Autodesk Inventor part; units mm, degrees
ref_plane "YZ Plane" through (0, 0, 0) normal (1, 0, 0) x (0, 1, 0)
ref_plane "XZ Plane" through (0, 0, 0) normal (0, 1, 0) x (-1, 0, 0)
ref_plane "XY Plane" through (0, 0, 0) normal (0, 0, 1) x (1, 0, 0)
sketch "Sketch1" plane through (0, 0, 0) normal (1, 0, 0) x (0, 1, 0)
  line L0 (-15.866, 25.4808) -> (14.134, -26.4808)
  line L1 (14.134, -26.4808) -> (15.866, -25.4808)
  line L2 (15.866, -25.4808) -> (-14.134, 26.4808)
  line L3 (-14.134, 26.4808) -> (-15.866, 25.4808)
  line L4 (-15.866, 25.4808) -> (15.866, -25.4808) construction
  line L5 (14.134, -26.4808) -> (-14.134, 26.4808) construction
  line L6 (-15.866, 25.4808) -> (44.134, 25.4808) construction
  point P0 (0, 0)
  dimension "d0" = 60
  dimension "d1" = 60
  dimension "d2" = 2
extrude "Extrusion1" add sketch "Sketch1" along normal blind 150
sketch "Sketch2" plane through (0, 0, 0) normal (0, 1, 0) x (-1, 0, 0)
  circle A0 centre (0, 0) radius 16.75
  dimension "d5" = 33.5
extrude "Extrusion2" cut sketch "Sketch2" along normal through all both and the other way through all
fillet "Fillet1" radius 2 4 edges at (150, -15, 25.9808) (150, 15, -25.9808) (0, -15, 25.9808) (0, 15, -25.9808)
equation "\"BendRadius\" = Thickness"
equation "\"BendReliefWidth\" = Thickness"
equation "\"BendReliefDepth\" = 0.5 * Thickness"
equation "\"CornerReliefSize\" = 4 * Thickness"
equation "\"MinimumRemnant\" = 2 * Thickness"
equation "\"TransitionRadius\" = BendRadius"
equation "\"JacobiRadiusSize\" = BendRadius"
equation "\"GapSize\" = Thickness"
properties part number "лопасть" material "Stainless Steel"
Model file for the job. Use its own axes, mm. Round coordinates to 2 decimals unless told otherwise and drop trailing zeros. Loops run counter-clockwise (first coordinate to the right, second up) from the corner with the lowest first, then second, coordinate; pieces in that order, holes last. Notation, with made-up numbers: (-16, 19.5) -> (27, 19.5) arc R21 ccw to (27, 49.5) -> close; hole circle Ø2 at (19.25, -21). An arc over 180 degrees is marked (long way). Answer as CSV lines item,"result". Start each with the question number.
1) Slice it at C-C (z = 22). List the corners of the cut face in (x, y), plus the area to 3 significant figures.
2) Slice it at B-B (x = 57). List the corners of the cut face in (y, z), plus the area to 3 significant figures.
3) Slice it at A-A (x = 13). List the corners of the cut face in (y, z), plus the area to 3 significant figures.
4) Probe line 1 along Z through (x, y) = (89, 14); line 2 along Z through (x, y) = (117, 13); line 3 along Y through (x, z) = (103, 10.5). List the from-to ranges inside material, lowest first.
5) Pin check, flat tips, straight feed: P1, Ø10, axis at x = 127.5, y = 6.5, coming from the -Z side; P2, Ø1.5, axis at y = 8, z = -12, coming from the -X side; P3, Ø3, axis at x = 78, z = 18, coming from the -Y side. Stop position of each tip, or through.
Filled in:
1,outline,"(0, -13.86) -> (150, -13.86) -> (150, -11.55) -> (0, -11.55) -> close"
1,area,"346 mm2"
2,outline,"(-15.87, 25.48) -> (14.13, -26.48) -> (15.87, -25.48) -> (-14.13, 26.48) -> close"
2,area,"120 mm2"
3,outline,"(-15.87, 25.48) -> (-7.25, 10.56) -> (-4.94, 10.56) -> (-14.13, 26.48) -> close; (4.94, -10.56) -> (14.13, -26.48) -> (15.87, -25.48) -> (7.25, -10.56) -> close"
3,area,"71.2 mm2"
4,line 1,"z = -26.25 to -22.25"
4,line 2,"z = -24.52 to -20.52"
4,line 3,"y = -7.22 to -4.91"
5,P1,"stops at z = -21.92"
5,P2,"stops at x = 10.86"
5,P3,"stops at y = -12.41"
